Read the model definition and answer for the solid it produces. Units are mm, in the model's axes. Face numbers are marked on the shaded views. A direction names the side the tool comes from. Give positions to 0.01 mm unless a question says otherwise; leave off trailing zeros. Loops run counter-clockwise (first coordinate to the right, second up) from the corner with the lowest first, then second, coordinate; pieces in that order, holes last. Notation, with made-up numbers: (-26, 40.5) -> (-16, 40.5) arc R21 ccw to (-16, 62.5) -> close; hole circle Ø11 at (18, 43). An arc over 180 degrees is marked (long way). One line per item, written item: value. Start each with the question number.
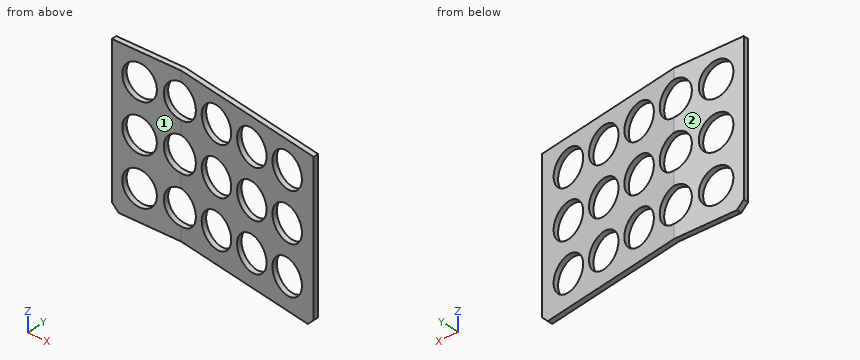
Autodesk Inventor part; units mm, degrees
ref_plane "Work Plane1" through (-25.2502, -11.5527, 0) normal (0, -1, 0) x (1, 0, 0)
ref_plane "YZ Plane" through (0, 0, 0) normal (1, 0, 0) x (0, 1, 0)
ref_plane "XZ Plane" through (0, 0, 0) normal (0, 1, 0) x (-1, 0, 0)
sketch "Sketch1" plane through (0, 0, 0) normal (0, 0, 1) x (1, 0, 0)
  line L0 (-25.2502, -1.5527) -> (-5.2502, -1.5527)
  line L1 (-5.2502, -1.5527) -> (39.7498, -9.4874)
  line L2 (-25.2502, -1.5527) -> (-25.2502, -0.0527)
  line L3 (-25.2502, -0.0527) -> (-5.1189, -0.0527)
  line L4 (-5.1189, -0.0527) -> (39.7498, -7.9642)
  line L5 (39.7498, -7.9642) -> (39.7498, -9.4874)
  point P0 (0, 0)
  dimension "d1" = 170
  dimension "d2" = 1.5
  dimension "d3" = 1.5
  dimension "d4" = 65
  dimension "d7" = 20
extrude "Extrusion1" add sketch "Sketch1" along normal blind 45
ref_plane "Work Plane1" through (-25.2502, -11.5527, 0) normal (0, -1, 0) x (1, 0, 0)
sketch "Sketch2" plane through (-25.2502, -11.5527, 0) normal (0, -1, 0) x (1, 0, 0)
  line L0 (20, 0) -> (65, 0)
  line L1 (65, 0) -> (65, 45)
  line L2 (20, 45) -> (65, 45)
  line L3 (20, 0) -> (20, 45)
  line L4 (0, 0) -> (20, 0)
  line L5 (20, 0) -> (20, 45)
  line L6 (0, 45) -> (20, 45)
  line L7 (0, 0) -> (0, 45)
  circle A0 centre (8, 37) radius 5
  circle A1 centre (8, 23) radius 5
  circle A2 centre (8, 9) radius 5
  circle A3 centre (20, 37) radius 5
  circle A4 centre (20, 23) radius 5
  circle A5 centre (20, 9) radius 5
  circle A6 centre (32, 37) radius 5
  circle A7 centre (32, 23) radius 5
  circle A8 centre (32, 9) radius 5
  circle A9 centre (44, 37) radius 5
  circle A10 centre (44, 23) radius 5
  circle A11 centre (44, 9) radius 5
  circle A12 centre (56, 37) radius 5
  circle A13 centre (56, 23) radius 5
  circle A14 centre (56, 9) radius 5
  point P0 (25.2502, 0)
  dimension "d9" = 10
  dimension "d10" = 8
  dimension "d11" = 8
  dimension "d14" = 14
  dimension "d17" = 12
extrude "Extrusion2" cut sketch "Sketch2" against normal through all contours A5 L3 | L3 A5 | A4 L3 | L3 A4 | A3 L3 | L3 A3 | A0 | A1 | A2 | A6 | A7 | A8 | A9 | A10 | A11 | A12 | A13 | A14
chamfer "Chamfer1" distance 2 angle 45 2 edges at (-25.2502, -0.8027, 0) (39.7498, -8.7258, 0)
equation "\"d3\" = d2"
equation "\"d11\" = d10"
properties part number "CNCM_ALU_Second_sieve" material "Aluminum 6061"
Item 1: Section D-D, the plane x = 19.5 is taken. Determine the outline of the cut face in (y, z).
Item 2: Consider L1, parallel to Y at x = -11, z = 32; L2, parallel to Z at x = -18, y = -1.5; L3, parallel to Y at x = 21.5, z = 15. Determine where each line is inside the solid, lowest interval first. Write a range as [from, to].
Item 3: Section A-A, the plane z = 13 is taken. Determine the outline of the cut face in (x, y).
Item 4: Section B-B, the plane x = -16 is taken. Determine the outline of the cut face in (y, z), plus the area to 3 significant figures.
Item 5: For the marked faces 1 and 2, determine the directions among +Z, -Z, +X, -X, +Y, -Y from which every point of the face is accessible in a straight line to the end or side of a thin tool.
Item 6: Flat-ended cylindrical pins translate along their axes: pin 1 (9 mm diameter, centred on x = -5.25, z = 37, fed in from -Y); pin 2 (6 mm diameter, centred on x = -18.5, z = 14.5, fed in from -Y); pin 3 (4 mm diameter, centred on x = 7.5, z = 14, fed in from -Y); pin 4 (16 mm diameter, centred on x = 30.75, z = 23, fed in from -Y). Find the tip coordinate at first contact, or state that the pin passes through.
Item 7: Section C-C, the plane z = 30 is taken. Determine the outline of the cut face in (x, y), plus the area to 3 significant figures.
Computed values:
1. outline: (-5.92, 0) -> (-4.39, 0) -> (-4.39, 4.06) -> (-5.92, 4.06) -> close; (-5.92, 13.94) -> (-4.39, 13.94) -> (-4.39, 18.06) -> (-5.92, 18.06) -> close; (-5.92, 27.94) -> (-4.39, 27.94) -> (-4.39, 32.06) -> (-5.92, 32.06) -> close; (-5.92, 41.94) -> (-4.39, 41.94) -> (-4.39, 45) -> (-5.92, 45) -> close
2. L1: [-1.55, -0.05]
2. L2: [0, 4.06], [13.94, 18.06], [27.94, 32.06], [41.94, 45]
2. L3: [-6.27, -4.75]
3. outline: (-25.25, -1.55) -> (-20.25, -1.55) -> (-20.25, -0.05) -> (-25.25, -0.05) -> close; (-14.25, -1.55) -> (-8.25, -1.55) -> (-8.25, -0.05) -> (-14.25, -0.05) -> close; (-2.25, -2.08) -> (3.75, -3.14) -> (3.75, -1.62) -> (-2.25, -0.56) -> close; (9.75, -4.2) -> (15.75, -5.26) -> (15.75, -3.73) -> (9.75, -2.67) -> close; (21.75, -6.31) -> (27.75, -7.37) -> (27.75, -5.85) -> (21.75, -4.79) -> close; (33.75, -8.43) -> (39.75, -9.49) -> (39.75, -7.96) -> (33.75, -6.91) -> close
4. outline: (-1.55, 0) -> (-0.05, 0) -> (-0.05, 4.16) -> (-1.55, 4.16) -> close; (-1.55, 13.84) -> (-0.05, 13.84) -> (-0.05, 18.16) -> (-1.55, 18.16) -> close; (-1.55, 27.84) -> (-0.05, 27.84) -> (-0.05, 32.16) -> (-1.55, 32.16) -> close; (-1.55, 41.84) -> (-0.05, 41.84) -> (-0.05, 45) -> (-1.55, 45) -> close
4. area: 23.9 mm²
5. face 1: +Z, -Z, -X, -Y
5. face 2: +Z, -Z, +X, -X, +Y
6. pin 1: through
6. pin 2: y = -1.55
6. pin 3: y = -4.15
6. pin 4: y = -9.31
7. outline: (-25.25, -1.55) -> (-5.25, -1.55) -> (39.75, -9.49) -> (39.75, -7.96) -> (-5.12, -0.05) -> (-25.25, -0.05) -> close
7. area: 98.5 mm²
